For this review, take the finished solid that the model builds, in its own axes (mm). Face numbers are marked on the shaded views. Give positions to 0.01 mm unless a question says otherwise; leave off trailing zeros. Order: outer loops, then holes, each group sorted by start corner. A loop starts at its lowest first (then second) coordinate and runs counter-clockwise, first axis right, second up.
Autodesk Inventor part; units mm, degrees
ref_plane "YZ Plane" through (0, 0, 0) normal (1, 0, 0) x (0, 1, 0)
ref_plane "XZ Plane" through (0, 0, 0) normal (0, 1, 0) x (-1, 0, 0)
ref_plane "XY Plane" through (0, 0, 0) normal (0, 0, 1) x (1, 0, 0)
sketch "Sketch1" plane through (0, 0, 0) normal (0, 1, 0) x (-1, 0, 0)
  line L0 (0, 0) -> (5, 0)
  line L1 (5, 0) -> (5, -34)
  line L2 (5, -34) -> (0, -34)
  line L3 (0, -34) -> (0, 0)
  dimension "d0" = 5
  dimension "d1" = 34
extrude "Extrusion1" add sketch "Sketch1" along normal blind 3
sketch "Sketch2" plane through (0, 3, 0) normal (0, 1, 0) x (1, 0, 0)
  line L0 (-5, 0) -> (0, 0)
  line L1 (-5, 34) -> (-5, 0)
  line L2 (0, 0) -> (-5, 0)
  line L3 (-5, 0) -> (-5, 3)
  line L4 (-5, 3) -> (0, 3)
  line L5 (0, 3) -> (0, 0)
  line L6 (0, 34) -> (-5, 34)
  line L7 (-5, 34) -> (0, 34)
  line L8 (0, 34) -> (0, 31)
  line L9 (0, 31) -> (-5, 31)
  line L10 (-5, 31) -> (-5, 34)
  dimension "d4" = 3
  dimension "d5" = 5
  dimension "d6" = 3
extrude "Extrusion2" add sketch "Sketch2" along normal blind 5
fillet "Fillet1" radius 2.5 4 edges at (0, 8, -1.5) (-5, 8, -1.5) (-5, 8, -32.5) (0, 8, -32.5)
sketch "Sketch3" plane through (-5, 3, -31) normal (0, 0, 1) x (1, 0, 0)
  point P0 (5, -3)
sketch "Sketch4" plane through (-5, 0, 0) normal (0, 0, 1) x (1, 0, 0)
  circle A0 centre (2.5, 5.5) radius 1
  arc A1 (5, 5.5) -> (0, 5.5) centre (2.5, 5.5) ccw
  line L0 (5, 0) -> (5, 5.5)
  dimension "d10" = 2
  dimension "d11" = 0
  dimension "d12" = 2.5
sketch "Sketch5" plane through (0, 0, -34) normal (0, 0, -1) x (-1, 0, 0)
  circle A0 centre (2.5, 5.5) radius 1
  arc A1 (5, 5.5) -> (0, 5.5) centre (2.5, 5.5) ccw
  line L0 (5, 0) -> (5, 5.5)
  point P0 (0, 0)
  dimension "d13" = 2
  dimension "d14" = 0
  dimension "d15" = 2.5
extrude "Extrusion3" cut sketch "Sketch5" against normal blind 3
extrude "Extrusion4" cut sketch "Sketch4" against normal blind 3
fillet "Fillet2" radius 0.5 20 edges at (-4.2679, 7.2679, -34) (-5, 2.7503, -34) (0, 2.7503, -34) (-4.2679, 7.2679, -31) (-5, 4.2503, -31) (0, 4.2503, -31) (0, 3, -17) (0, 0, -17) (-2.5, 0, -34) (-0.7321, 7.2679, -3) (-5, 4.2503, -3) (0, 4.2503, -3) (-0.7321, 7.2679, 0) (-5, 2.7503, 0) (0, 2.7503, 0) (-2.5, 3, -3) (-5, 3, -17) (-5, 0, -17) (-2.5, 0, 0) (-2.5, 3, -31)
properties part number "support"
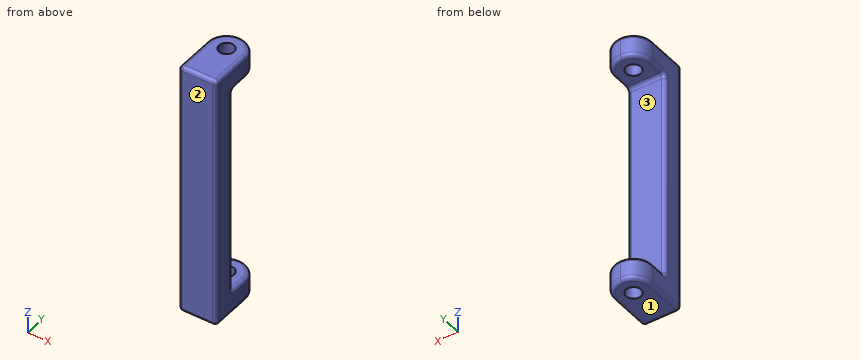
1) Draft analysis for pull direction Z (two halves, no side actions). For the marked faces 1, 2 and 3, state which applies: +Z half, -Z half, draft (parallel to the pull), parting line (faces both ways), or undercut.
Answer sheet:
face 1: -Z half
face 2: draft
face 3: undercut
2) We need section A-A on y = 4. Give the boundary of the cut face in (x, z), then the cut area to 3 significant figures.
Answer sheet:
outline: (-5, -33.5) arc R0.5 ccw to (-4.5, -34) - (-0.5, -34) arc R0.5 ccw to (0, -33.5) - (0, -31.5) arc R0.5 ccw to (-0.5, -31) - (-4.5, -31) arc R0.5 ccw to (-5, -31.5) - close; (-5, -2.5) arc R0.5 ccw to (-4.5, -3) - (-0.5, -3) arc R0.5 ccw to (0, -2.5) - (0, -0.5) arc R0.5 ccw to (-0.5, 0) - (-4.5, 0) arc R0.5 ccw to (-5, -0.5) - close
area: 29.6 mm2
3) Clearance check with flat-ended pins moving along their axes: pin 1 (3 mm diameter, centred on x = -2.5, z = -22.5, fed in from +Y); pin 2 (1.6 mm diameter, centred on x = -2.5, y = 5.5, fed in from -Z). State where each tip first meets the part, or that it passes through.
Answer sheet:
pin 1: stops at y = 3
pin 2: passes through
4) To check wall thickness, follow line 1 (Z direction, x = -1.2, y = 4.25); line 2 (Y direction, x = -2.5, z = -1.85); line 3 (Y direction, x = -3.3, z = -26.5). State the ranges of each line that lie inside material, in increasing order.
Answer sheet:
line 1: z = -34 to -31, -3 to 0
line 2: y = 0 to 4.5, 6.5 to 8
line 3: y = 0 to 3
5) We need section B-B on z = -22.5. Give the boundary of the cut face in (x, y), then the cut area to 3 significant figures.
Answer sheet:
outline: (-5, 0.5) arc R0.5 ccw to (-4.5, 0) - (-0.5, 0) arc R0.5 ccw to (0, 0.5) - (0, 2.5) arc R0.5 ccw to (-0.5, 3) - (-4.5, 3) arc R0.5 ccw to (-5, 2.5) - close
area: 14.8 mm2
6) We need section C-C on x = -3.05. Count the separate pieces of the cut face and the enclosed holes in it, then the cut area to 3 significant figures.
Answer sheet:
separate pieces: 3
enclosed holes: 0
area: 121 mm2
